```python
from build123d import *

# Parameters (mm, degrees)
BOSS_EXTRUDE1_DEPTH = 5
SKETCH2_W           = 113
SKETCH2_H           = 72
BOSS_EXTRUDE2_DEPTH = 25
SKETCH3_R           = 1.25
CUT_EXTRUDE1_DEPTH  = 6
SKETCH4_W           = 30
SKETCH4_H           = 28.6
BOSS_EXTRUDE3_DEPTH = 3
SKETCH5_W           = 10
SKETCH5_H           = 3
BOSS_EXTRUDE4_DEPTH = 12.4
SKETCH6_R           = 1
CUT_EXTRUDE2_DEPTH  = 4
SKETCH12_W          = 8
SKETCH12_H          = 5
CUT_EXTRUDE3_DEPTH  = 21


with BuildPart() as part:
    # Sketch1 → Boss-Extrude1 (new body)
    with BuildSketch(Plane(origin=(0, 0, 0), x_dir=(1, 0, 0), z_dir=(0, 1, 0))):
        Polygon((-42.5, -81), (-42.5, 29), (-60.5, 29), (-60.5, 109), (60.5, 109), (60.5, 29), (42.5, 29), (42.5, -81), (37.5, -81), (37.5, 29), (-37.5, 29), (-37.5, -81), align=None)
    extrude(amount=BOSS_EXTRUDE1_DEPTH)

    # Sketch2 → Boss-Extrude2 (add)
    with BuildSketch(Plane(origin=(0, 5, 0), x_dir=(1, 0, 0), z_dir=(0, 1, 0))):
        Polygon((-60.5, 109), (-60.5, 29), (-42.5, 29), (-37.5, 29), (37.5, 29), (42.5, 29), (60.5, 29), (60.5, 109), align=None)
        with Locations((0, 69)):
            Rectangle(SKETCH2_W, SKETCH2_H, mode=Mode.SUBTRACT)
    extrude(amount=BOSS_EXTRUDE2_DEPTH)

    # Sketch3 → Cut-Extrude1 (cut)
    with BuildSketch(Plane(origin=(0, 30, 0), x_dir=(1, 0, 0), z_dir=(0, 1, 0))):
        with Locations(Location((-58.5, 31, 0), (0, 0, 270))):
            Circle(SKETCH3_R)
        with Locations(Location((58.5, 31, 0), (0, 0, 90))):
            Circle(SKETCH3_R)
        with Locations(Location((-58.5, 107, 0), (0, 0, 90))):
            Circle(SKETCH3_R)
        with Locations(Location((58.5, 107, 0), (0, 0, 270))):
            Circle(SKETCH3_R)
    extrude(amount=-CUT_EXTRUDE1_DEPTH, mode=Mode.SUBTRACT)

    # Sketch4 → Boss-Extrude3 (add)
    with BuildSketch(Plane(origin=(0, 5, 0), x_dir=(1, 0, 0), z_dir=(0, 1, 0))):
        with Locations((27.5, -36)):
            Rectangle(SKETCH4_W, SKETCH4_H)
    extrude(amount=BOSS_EXTRUDE3_DEPTH)

    # Sketch5 → Boss-Extrude4 (add)
    with BuildSketch(Plane(origin=(0, 8, 0), x_dir=(1, 0, 0), z_dir=(0, 1, 0))):
        with Locations((17.5, -23.2)):
            Rectangle(SKETCH5_W, SKETCH5_H)
        with Locations((17.5, -48.8)):
            Rectangle(SKETCH5_W, SKETCH5_H)
    extrude(amount=BOSS_EXTRUDE4_DEPTH)

    # Sketch6 → Cut-Extrude2 (cut)
    with BuildSketch(Plane(origin=(0, 20.4, 0), x_dir=(1, 0, 0), z_dir=(0, 1, 0))):
        with Locations(Location((17.5, -48.8, 0), (0, 0, 270))):
            Circle(SKETCH6_R)
        with Locations(Location((17.5, -23.2, 0), (0, 0, 270))):
            Circle(SKETCH6_R)
    extrude(amount=-CUT_EXTRUDE2_DEPTH, mode=Mode.SUBTRACT)

    # Sketch12 → Cut-Extrude3 (cut)
    with BuildSketch(Plane.XY.offset(-29)):
        with Locations((0, 10)):
            Rectangle(SKETCH12_W, SKETCH12_H)
    extrude(amount=-CUT_EXTRUDE3_DEPTH, mode=Mode.SUBTRACT)


solid = part.part
```
Can you work these out from the model? Positions are in its coordinate system, mm. A direction names the side the tool comes from. Coordinates: 2 decimals unless noted, no trailing zeros. Loops run counter-clockwise (first coordinate to the right, second up) from the corner with the lowest first, then second, coordinate; pieces in that order, holes last.
Item 1: Which directions (+Z, -Z, +X, -X, +Y, -Y) give clear straight access to the entire face, cutting with the end or side of a thin tool? Please do faces 1 (the face through (4, 10, -31)), 2 (the face through (17, 14, 24.7)), 3 (the face through (37.5, 2, 27)).
Answers below:
face 1: +Z
face 2: +X, -X, +Y
face 3: +Z, -Y
Item 2: If we mould it in two halves opening along Z, with no side actions, what happens to faces 4 (the face through (21, 11, 50.3)), 5 (the face through (56.5, 17, -68)), 6 (the face through (40, 5, 65))? For each: released by +Z, released by -Z, zero draft, split by the parting line, or undercut.
Answers below:
face 4: released by +Z
face 5: undercut
face 6: zero draft
Item 3: Suppose I cut it at C-C (z = -90). Please give me the cut outline in (x, y), then the cut area to 3 significant figures.
Answers below:
outline: (-60.5, 0) - (60.5, 0) - (60.5, 30) - (56.5, 30) - (56.5, 5) - (-56.5, 5) - (-56.5, 30) - (-60.5, 30) - close
area: 805 mm2
Item 4: Suppose I cut it at B-B (z = 31.5). Please give me the cut outline in (x, y), then the cut area to 3 significant figures.
Answers below:
outline: (-42.5, 0) - (-37.5, 0) - (-37.5, 5) - (-42.5, 5) - close; (12.5, 5) - (37.5, 5) - (37.5, 0) - (42.5, 0) - (42.5, 8) - (12.5, 8) - close
area: 140 mm2
Item 5: Suppose I cut it at D-D (x = -48). Please give me the cut outline in (y, z).
Answers below:
outline: (0, -109) - (30, -109) - (30, -105) - (5, -105) - (5, -33) - (30, -33) - (30, -29) - (0, -29) - close
Item 6: Suppose I cut it at A-A (x = 20.5). Please give me the cut outline in (y, z), then the cut area to 3 significant figures.
Answers below:
outline: (0, -109) - (30, -109) - (30, -105) - (5, -105) - (5, -33) - (30, -33) - (30, -29) - (0, -29) - close; (5, 21.7) - (20.4, 21.7) - (20.4, 24.7) - (8, 24.7) - (8, 47.3) - (20.4, 47.3) - (20.4, 50.3) - (5, 50.3) - close
area: 760 mm2
Item 7: Please list where these lines run through material, in increasing order: L1, parallel to X at y = 28.45, z = -31; L2, parallel to Z at x = -5, y = 15; L3, parallel to X at y = 19.15, z = 23.2.
Answers below:
L1: x = -60.5 to -59.75, -57.25 to 57.25, 59.75 to 60.5
L2: z = -109 to -105, -33 to -29
L3: x = 12.5 to 16.5, 18.5 to 22.5
Item 8: I'm going to push flat-ended pins straight in: pin 1 (3 mm diameter, centred on x = -59, z = -106.5, fed in from +Y); pin 2 (6 mm diameter, centred on x = -29.5, y = 23, fed in from +Z); pin 3 (5 mm diameter, centred on x = 18.5, y = 16.5, fed in from +Z); pin 4 (1.6 mm diameter, centred on x = 18, z = 48.5, fed in from +Y). Where does each tip first touch, or does it pass through?
Answers below:
pin 1: stops at y = 30
pin 2: stops at z = -29
pin 3: stops at z = 50.3
pin 4: stops at y = 20.4
